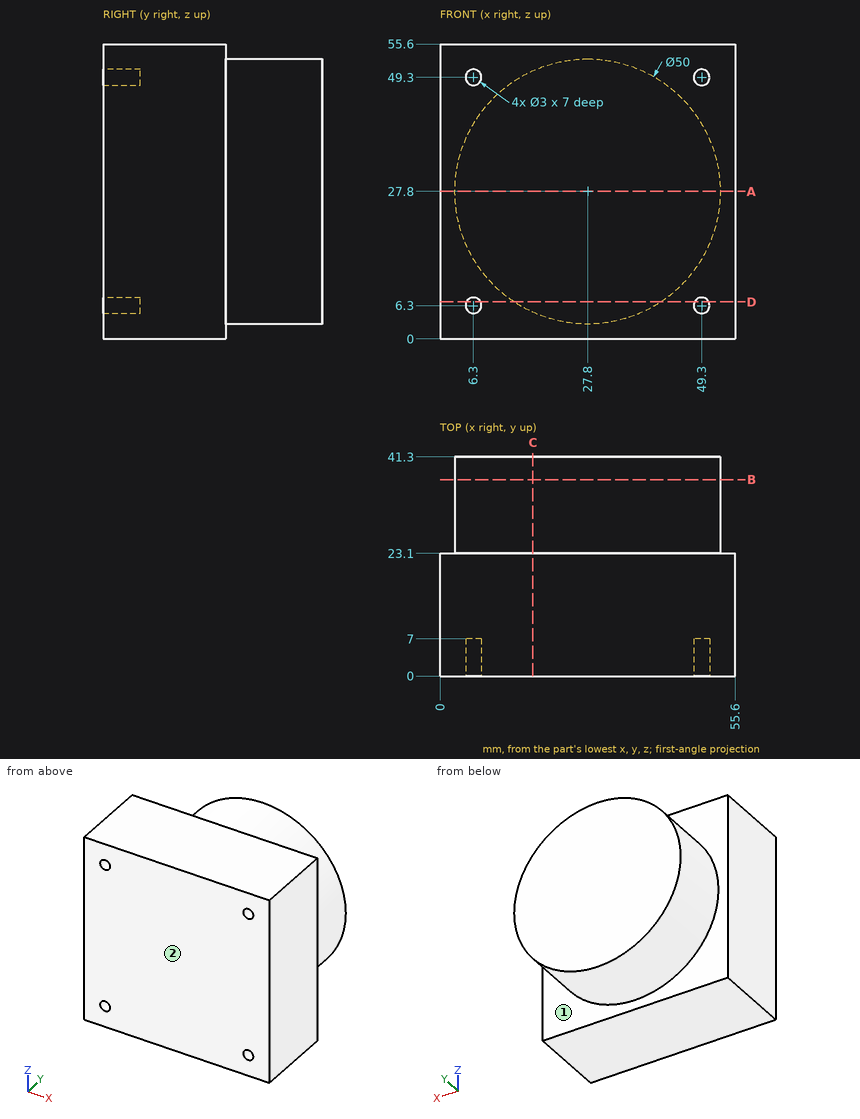
Answer from the drawing. Dimensions are ordinates in mm from the lowest x, y and z of the part. A direction names the side the tool comes from. Coordinates: 2 decimals unless noted, no trailing zeros. Order: outer loops, then holes, each group sorted by start corner. A loop starts at its lowest first (then second) coordinate and runs counter-clockwise, first axis right, second up. Notation, with made-up numbers: (53.5, -34) - (108.5, -34) arc R35 cw to (108.5, 0) - close; hole circle Ø1 at (1, -14). An arc over 180 degrees is marked (long way). Answer as a JSON object with one key per item and string values. Group by question number.
Item 1: Section B-B (y = 37) is taken. Give the vertices of the cut face in (x, z).
Item 2: A tool of negligible diameter and unlimited length cuts with its end or side. For the marked faces 1 and 2, from which of +Z, -Z, +X, -X, +Y, -Y can it reach the whole face along a straight path? Write none if from no direction.
Item 3: Flat-ended cylindrical pins translate along their axes: P1, Ø6, axis at x = 23.5, z = 9.5, coming from the -Y side; P2, Ø0.9, axis at x = 48.5, z = 6, coming from the -Y side; P3, Ø5, axis at x = 49.3, z = 49.3, coming from the +Y side. Find the tip coordinate at first contact, or state that the pin passes through.
Item 4: Section D-D (z = 7) is taken. Give the vertices of the cut face in (x, y), plus the area to 3 significant figures.
Item 5: Section C-C (x = 17.5) is taken. Give the vertices of the cut face in (y, z), plus the area to 3 significant figures.
Item 6: Consider probe 1 along X at (y, z) = (3.5, 6.3); probe 2 along Z at (x, y) = (6, 3); probe 3 along Y at (x, z) = (8.5, 50). Determine where each line is inside the solid, lowest interval first. Write a range as from..to.
Item 7: Section A-A (z = 27.8) is taken. Give the vertices of the cut face in (x, y), plus the area to 3 significant figures.
Results are:
{
 "1": {"outline": "circle Ø50 at (27.8, 27.8)"},
 "2": {"face 1": "+Y", "face 2": "+Z, -Z, +X, -X, -Y"},
 "3": {"P1": "stops at y = 0", "P2": "stops at y = 7", "P3": "stops at y = 23.1"},
 "4": {"outline": "(0, 0) - (4.97, 0) - (4.97, 7) - (7.63, 7) - (7.63, 0) - (47.97, 0) - (47.97, 7) - (50.63, 7) - (50.63, 0) - (55.6, 0) - (55.6, 23.1) - (41.67, 23.1) - (41.67, 41.3) - (13.93, 41.3) - (13.93, 23.1) - (0, 23.1) - close", "area": "1,750 mm^2"},
 "5": {"outline": "(0, 0) - (23.1, 0) - (23.1, 5.02) - (41.3, 5.02) - (41.3, 50.58) - (23.1, 50.58) - (23.1, 55.6) - (0, 55.6) - close", "area": "2,110 mm^2"},
 "6": {"probe 1": "x = 0..4.8, 7.8..47.8, 50.8..55.6", "probe 2": "z = 0..4.83, 7.77..47.83, 50.77..55.6", "probe 3": "y = 0..23.1"},
 "7": {"outline": "(0, 0) - (55.6, 0) - (55.6, 23.1) - (52.8, 23.1) - (52.8, 41.3) - (2.8, 41.3) - (2.8, 23.1) - (0, 23.1) - close", "area": "2,190 mm^2"}
}
